The listing builds one solid part. Answer for the finished solid, in the listing's coordinates (mm). Face numbers are marked on the shaded views. A direction names the side the tool comes from. Coordinates: 2 decimals unless noted, no trailing zeros. Order: outer loops, then holes, each group sorted by start corner. A loop starts at its lowest first (then second) coordinate and runs counter-clockwise, first axis right, second up. Notation, with made-up numbers: M 84,0 L 112,0 A19 cw 112,32 Z; hole C 12,-30 d6. An arc over 180 degrees is marked long. One line per item, written item: value. Start each with the question number.
Q1. For the marked faces 1 and 2, determine the directions among +Z, -Z, +X, -X, +Y, -Y from which every point of the face is accessible in a straight line to the end or side of a thin tool.
Q2. The part is cut by section D-D on y = 18.5. Give the vertices of the cut face in (x, z).
Q3. The part is cut by section C-C on z = -6.5. Give the vertices of the cut face in (x, y), then the cut area to 3 significant figures.
Q4. Straight lines are drawn through the part: line 1 along X through (y, z) = (31.15, -16.5); line 2 along Z through (x, y) = (39, 20); line 3 along Z through (x, y) = (27, 31). For each, find the intervals that lie inside material, in ascending order. Write a range as [from, to].
Q5. The part is cut by section B-B on y = 26.5. Give the vertices of the cut face in (x, z), then the cut area to 3 significant figures.
Q6. Each of these flat-tipped pins is pushed along its axis until it touches: pin 1 Ø3.5 at (x, z) = (28, 1) entering from -Y; pin 2 Ø3.5 at (y, z) = (20.5, -35) entering from -X; pin 3 Ø1.5 at (y, z) = (31, -32) entering from -X; pin 4 Ø3.5 at (x, z) = (34.57, -23.57) entering from -Y. Where does it stop, or does it pass through?
Q7. The part is cut by section A-A on x = 27.5. Give the vertices of the cut face in (y, z).
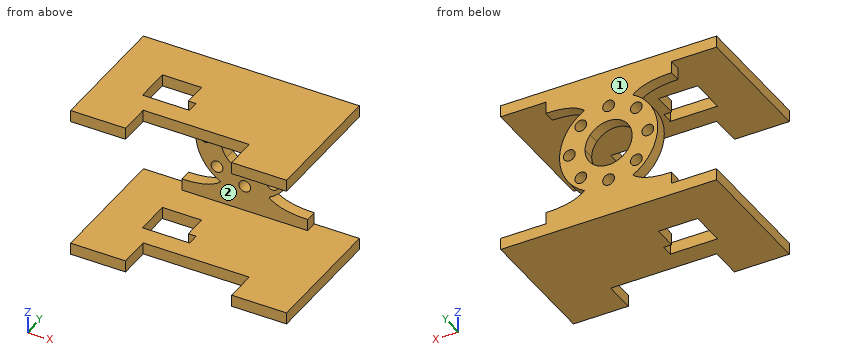
```python
from build123d import *

# Parameters (mm, degrees)
ESQUISSE1_W                = 55
ESQUISSE1_H                = 33
BOSS_EXTRU_1_DEPTH         = 3
ENL_V_MAT_EXTRU_1_REACH    = 66.211
ENL_V_MAT_EXTRU_2_REACH    = 66.211
ESQUISSE4_W                = 32
ESQUISSE4_H                = 3
BOSS_EXTRU_2_DEPTH         = 3
ENL_V_MAT_EXTRU_3_REACH    = 74.132
ESQUISSE5_R                = 1.5
R_P_TITION_LIN_AIRE1_COUNT = 2
R_P_TITION_LIN_AIRE1_PITCH = 36


with BuildPart() as part:
    # Esquisse1 → Boss.-Extru.1 (new body)
    with BuildSketch(Plane.XY):
        with Locations((27.5, 16.5)):
            Rectangle(ESQUISSE1_W, ESQUISSE1_H)
    boss_extru_1 = extrude(amount=BOSS_EXTRU_1_DEPTH)

    # Esquisse2 → Enlèv. mat.-Extru.1 (cut, up to next)
    with BuildSketch(Plane.XY.offset(3), mode=Mode.PRIVATE) as enl_v_mat_extru_1_sk1:
        Polygon((27.5, 8), (41, 8), (41, 0), (14, 0), (14, 8), align=None)
    enl_v_mat_extru_1_tool1 = extrude(enl_v_mat_extru_1_sk1.sketch, amount=-ENL_V_MAT_EXTRU_1_REACH, mode=Mode.PRIVATE) & part.part
    enl_v_mat_extru_1 = enl_v_mat_extru_1_tool1.solids().sort_by_distance((27.5, 4, 3))[0]
    add(enl_v_mat_extru_1, mode=Mode.SUBTRACT)

    # Esquisse3 → Enlèv. mat.-Extru.2 (cut, up to next)
    with BuildSketch(Plane.XY.offset(3), mode=Mode.PRIVATE) as enl_v_mat_extru_2_sk1:
        Polygon((11, 22), (21, 22), (21, 16), (23, 16), (23, 13), (11, 13), (11, 16), align=None)
    enl_v_mat_extru_2_tool1 = extrude(enl_v_mat_extru_2_sk1.sketch, amount=-ENL_V_MAT_EXTRU_2_REACH, mode=Mode.PRIVATE) & part.part
    enl_v_mat_extru_2 = enl_v_mat_extru_2_tool1.solids().sort_by_distance((16.375, 17.3125, 3))[0]
    add(enl_v_mat_extru_2, mode=Mode.SUBTRACT)

    # Esquisse4 → Boss.-Extru.2 (add)
    with BuildSketch(Plane(origin=(0, 33, 0), x_dir=(1, 0, 0), z_dir=(0, 1, 0))):
        Polygon((11.5, 0), (27.5, 0), (43.5, 0), (43.5, 3), (11.5, 3), align=None)
        with BuildLine():
            add(Edge.make_bspline(
                [(11.5, 3), (18.557221365, 3), (21.334379392, 5.626402504)],
                knots=[0, 0, 0, 0.441076335, 0.441076335, 0.441076335], degree=2))
            Line((11.5, 3), (43.5, 3))
            add(Edge.make_bspline(
                [(43.5, 3), (36.442778635, 3), (33.665620608, 5.626402504)],
                knots=[0, 0, 0, 0.441076335, 0.441076335, 0.441076335], degree=2))
            ThreePointArc((33.665620608, 5.626402504), (27.5, 4), (21.334379392, 5.626402504))
        make_face()
        with BuildLine():
            add(Edge.make_bspline(
                [(21.334379392, 5.626402504), (23.913128098, 8.065166158), (22.80153106, 12.768460155)],
                knots=[0.441076335, 0.441076335, 0.441076335, 0.850640724, 0.850640724, 0.850640724], degree=2))
            ThreePointArc((21.334379392, 5.626402504), (27.5, 4), (33.665620608, 5.626402504))
            add(Edge.make_bspline(
                [(33.665620608, 5.626402504), (31.086871902, 8.065166158), (32.19846894, 12.768460155)],
                knots=[0.441076335, 0.441076335, 0.441076335, 0.850640724, 0.850640724, 0.850640724], degree=2))
            ThreePointArc((32.19846894, 12.768460155), (27.5, 10.5), (22.80153106, 12.768460155))
        make_face()
        with BuildLine():
            add(Edge.make_bspline(
                [(33.665620608, 5.626402504), (31.086871902, 8.065166158), (32.19846894, 12.768460155)],
                knots=[0.441076335, 0.441076335, 0.441076335, 0.850640724, 0.850640724, 0.850640724], degree=2))
            ThreePointArc((33.665620608, 5.626402504), (38.300931849, 10.207951749), (40, 16.5))
            ThreePointArc((40, 16.5), (38.300931849, 22.792048251), (33.665620608, 27.373597496))
            add(Edge.make_bspline(
                [(33.665620608, 27.373597496), (31.086871902, 24.934833842), (32.19846894, 20.231539845)],
                knots=[0.441076335, 0.441076335, 0.441076335, 0.850640724, 0.850640724, 0.850640724], degree=2))
            ThreePointArc((32.19846894, 20.231539845), (33.165280825, 18.476004347), (33.5, 16.5))
            ThreePointArc((33.5, 16.5), (33.165280825, 14.523995653), (32.19846894, 12.768460155))
        make_face()
        with BuildLine():
            ThreePointArc((21.334379392, 27.373597496), (15, 16.5), (21.334379392, 5.626402504))
            add(Edge.make_bspline(
                [(21.334379392, 5.626402504), (23.913128098, 8.065166158), (22.80153106, 12.768460155)],
                knots=[0.441076335, 0.441076335, 0.441076335, 0.850640724, 0.850640724, 0.850640724], degree=2))
            ThreePointArc((22.80153106, 12.768460155), (21.834719175, 14.523995653), (21.5, 16.5))
            ThreePointArc((21.5, 16.5), (21.834719175, 18.476004347), (22.80153106, 20.231539845))
            add(Edge.make_bspline(
                [(21.334379392, 27.373597496), (23.913128098, 24.934833842), (22.80153106, 20.231539845)],
                knots=[0.441076335, 0.441076335, 0.441076335, 0.850640724, 0.850640724, 0.850640724], degree=2))
        make_face()
        with BuildLine():
            ThreePointArc((33.665620608, 27.373597496), (27.5, 29), (21.334379392, 27.373597496))
            add(Edge.make_bspline(
                [(21.334379392, 27.373597496), (23.913128098, 24.934833842), (22.80153106, 20.231539845)],
                knots=[0.441076335, 0.441076335, 0.441076335, 0.850640724, 0.850640724, 0.850640724], degree=2))
            ThreePointArc((22.80153106, 20.231539845), (27.5, 22.5), (32.19846894, 20.231539845))
            add(Edge.make_bspline(
                [(33.665620608, 27.373597496), (31.086871902, 24.934833842), (32.19846894, 20.231539845)],
                knots=[0.441076335, 0.441076335, 0.441076335, 0.850640724, 0.850640724, 0.850640724], degree=2))
        make_face()
        with BuildLine():
            add(Edge.make_bspline(
                [(11.5, 30), (18.557221365, 30), (21.334379392, 27.373597496)],
                knots=[0, 0, 0, 0.441076335, 0.441076335, 0.441076335], degree=2))
            ThreePointArc((21.334379392, 27.373597496), (27.5, 29), (33.665620608, 27.373597496))
            add(Edge.make_bspline(
                [(43.5, 30), (36.442778635, 30), (33.665620608, 27.373597496)],
                knots=[0, 0, 0, 0.441076335, 0.441076335, 0.441076335], degree=2))
            Line((43.5, 30), (11.5, 30))
        make_face()
        with Locations((27.5, 31.5)):
            Rectangle(ESQUISSE4_W, ESQUISSE4_H)
    extrude(amount=-BOSS_EXTRU_2_DEPTH)

    # Esquisse5 → Enlèv. mat.-Extru.3 (cut, up to next)
    with BuildSketch(Plane(origin=(0, 33, 0), x_dir=(1, 0, 0), z_dir=(0, 1, 0)), mode=Mode.PRIVATE) as enl_v_mat_extru_3_sk1:
        with Locations(Location((27.5, 26.5, 0), (0, 0, 270))):
            Circle(ESQUISSE5_R)
    enl_v_mat_extru_3_tool1 = extrude(enl_v_mat_extru_3_sk1.sketch, amount=-ENL_V_MAT_EXTRU_3_REACH, mode=Mode.PRIVATE) & part.part
    # Esquisse5 → Enlèv. mat.-Extru.3 (cut, up to next)
    with BuildSketch(Plane(origin=(0, 33, 0), x_dir=(1, 0, 0), z_dir=(0, 1, 0)), mode=Mode.PRIVATE) as enl_v_mat_extru_3_sk2:
        with Locations(Location((20.428932188, 23.571067812, 0), (0, 0, 270))):
            Circle(ESQUISSE5_R)
    enl_v_mat_extru_3_tool2 = extrude(enl_v_mat_extru_3_sk2.sketch, amount=-ENL_V_MAT_EXTRU_3_REACH, mode=Mode.PRIVATE) & part.part
    # Esquisse5 → Enlèv. mat.-Extru.3 (cut, up to next)
    with BuildSketch(Plane(origin=(0, 33, 0), x_dir=(1, 0, 0), z_dir=(0, 1, 0)), mode=Mode.PRIVATE) as enl_v_mat_extru_3_sk3:
        with Locations(Location((17.5, 16.5, 0), (0, 0, 270))):
            Circle(ESQUISSE5_R)
    enl_v_mat_extru_3_tool3 = extrude(enl_v_mat_extru_3_sk3.sketch, amount=-ENL_V_MAT_EXTRU_3_REACH, mode=Mode.PRIVATE) & part.part
    # Esquisse5 → Enlèv. mat.-Extru.3 (cut, up to next)
    with BuildSketch(Plane(origin=(0, 33, 0), x_dir=(1, 0, 0), z_dir=(0, 1, 0)), mode=Mode.PRIVATE) as enl_v_mat_extru_3_sk4:
        with Locations(Location((27.5, 6.5, 0), (0, 0, 270))):
            Circle(ESQUISSE5_R)
    enl_v_mat_extru_3_tool4 = extrude(enl_v_mat_extru_3_sk4.sketch, amount=-ENL_V_MAT_EXTRU_3_REACH, mode=Mode.PRIVATE) & part.part
    # Esquisse5 → Enlèv. mat.-Extru.3 (cut, up to next)
    with BuildSketch(Plane(origin=(0, 33, 0), x_dir=(1, 0, 0), z_dir=(0, 1, 0)), mode=Mode.PRIVATE) as enl_v_mat_extru_3_sk5:
        with Locations(Location((34.571067812, 9.428932188, 0), (0, 0, 270))):
            Circle(ESQUISSE5_R)
    enl_v_mat_extru_3_tool5 = extrude(enl_v_mat_extru_3_sk5.sketch, amount=-ENL_V_MAT_EXTRU_3_REACH, mode=Mode.PRIVATE) & part.part
    # Esquisse5 → Enlèv. mat.-Extru.3 (cut, up to next)
    with BuildSketch(Plane(origin=(0, 33, 0), x_dir=(1, 0, 0), z_dir=(0, 1, 0)), mode=Mode.PRIVATE) as enl_v_mat_extru_3_sk6:
        with Locations(Location((37.5, 16.5, 0), (0, 0, 270))):
            Circle(ESQUISSE5_R)
    enl_v_mat_extru_3_tool6 = extrude(enl_v_mat_extru_3_sk6.sketch, amount=-ENL_V_MAT_EXTRU_3_REACH, mode=Mode.PRIVATE) & part.part
    # Esquisse5 → Enlèv. mat.-Extru.3 (cut, up to next)
    with BuildSketch(Plane(origin=(0, 33, 0), x_dir=(1, 0, 0), z_dir=(0, 1, 0)), mode=Mode.PRIVATE) as enl_v_mat_extru_3_sk7:
        with Locations(Location((34.571067812, 23.571067812, 0), (0, 0, 270))):
            Circle(ESQUISSE5_R)
    enl_v_mat_extru_3_tool7 = extrude(enl_v_mat_extru_3_sk7.sketch, amount=-ENL_V_MAT_EXTRU_3_REACH, mode=Mode.PRIVATE) & part.part
    # Esquisse5 → Enlèv. mat.-Extru.3 (cut, up to next)
    with BuildSketch(Plane(origin=(0, 33, 0), x_dir=(1, 0, 0), z_dir=(0, 1, 0)), mode=Mode.PRIVATE) as enl_v_mat_extru_3_sk8:
        with Locations(Location((20.428932188, 9.428932188, 0), (0, 0, 270))):
            Circle(ESQUISSE5_R)
    enl_v_mat_extru_3_tool8 = extrude(enl_v_mat_extru_3_sk8.sketch, amount=-ENL_V_MAT_EXTRU_3_REACH, mode=Mode.PRIVATE) & part.part
    add(enl_v_mat_extru_3_tool1.solids().sort_by_distance((27.5, 33, -26.5))[0], mode=Mode.SUBTRACT)
    add(enl_v_mat_extru_3_tool2.solids().sort_by_distance((20.428932, 33, -23.571068))[0], mode=Mode.SUBTRACT)
    add(enl_v_mat_extru_3_tool3.solids().sort_by_distance((17.5, 33, -16.5))[0], mode=Mode.SUBTRACT)
    add(enl_v_mat_extru_3_tool4.solids().sort_by_distance((27.5, 33, -6.5))[0], mode=Mode.SUBTRACT)
    add(enl_v_mat_extru_3_tool5.solids().sort_by_distance((34.571068, 33, -9.428932))[0], mode=Mode.SUBTRACT)
    add(enl_v_mat_extru_3_tool6.solids().sort_by_distance((37.5, 33, -16.5))[0], mode=Mode.SUBTRACT)
    add(enl_v_mat_extru_3_tool7.solids().sort_by_distance((34.571068, 33, -23.571068))[0], mode=Mode.SUBTRACT)
    add(enl_v_mat_extru_3_tool8.solids().sort_by_distance((20.428932, 33, -9.428932))[0], mode=Mode.SUBTRACT)

    # Répétition linéaire1: Boss.-Extru.1, Enlèv. mat.-Extru.1, Enlèv. mat.-Extru.2 ×2
    with Locations(*[(0, 0, -i * R_P_TITION_LIN_AIRE1_PITCH) for i in range(1, R_P_TITION_LIN_AIRE1_COUNT)]):
        add(boss_extru_1)
        add(enl_v_mat_extru_1, mode=Mode.SUBTRACT)
        add(enl_v_mat_extru_2, mode=Mode.SUBTRACT)


solid = part.part
```
Output:
1. face 1: +Z, -Z, +X, -X, +Y
1. face 2: +X, -X, -Y
2. outline: M 0,-36 L 11,-36 L 11,-33 L 0,-33 Z; M 0,0 L 11,0 L 11,3 L 0,3 Z; M 21,-36 L 55,-36 L 55,-33 L 21,-33 Z; M 21,0 L 55,0 L 55,3 L 21,3 Z
3. outline: M 20,30 L 26,30 L 26,33 L 20,33 Z; M 29,30 L 35,30 L 35,33 L 29,33 Z
3. area: 36.0 mm^2
4. line 1: x = [15, 16], [19, 21.5], [33.5, 36], [39, 40]
4. line 2: z = [-36, -33], [0, 3]
4. line 3: z = [-36, -27.91], [-25.09, -22.48], [-10.52, -7.91], [-5.09, 3]
5. outline: M 0,-36 L 55,-36 L 55,-33 L 0,-33 Z; M 0,0 L 55,0 L 55,3 L 0,3 Z
5. area: 330 mm^2
6. pin 1: stops at y = 8
6. pin 2: stops at x = 0
6. pin 3: stops at x = 11.5
6. pin 4: stops at y = 30
7. outline: M 8,-36 L 33,-36 L 33,-28 L 30,-28 L 30,-33 L 8,-33 Z; M 8,0 L 30,0 L 30,-5 L 33,-5 L 33,3 L 8,3 Z; M 30,-25 L 33,-25 L 33,-22.5 L 30,-22.5 Z; M 30,-10.5 L 33,-10.5 L 33,-8 L 30,-8 Z
